Verification items for the finished model (mm, model axes). Face numbers are marked on the shaded views. A direction names the side the tool comes from. Give positions to 0.01 mm unless a question says otherwise; leave off trailing zeros. Loops run counter-clockwise (first coordinate to the right, second up) from the corner with the lowest first, then second, coordinate; pieces in that order, holes last. Notation, with made-up numbers: (43.25, -31.75) - (72.25, -31.75) arc R25 ccw to (72.25, 7.25) - close; hole circle Ø10 at (-8, -1). An arc over 180 degrees is marked (long way). Answer in a Markdown table with one row per item.
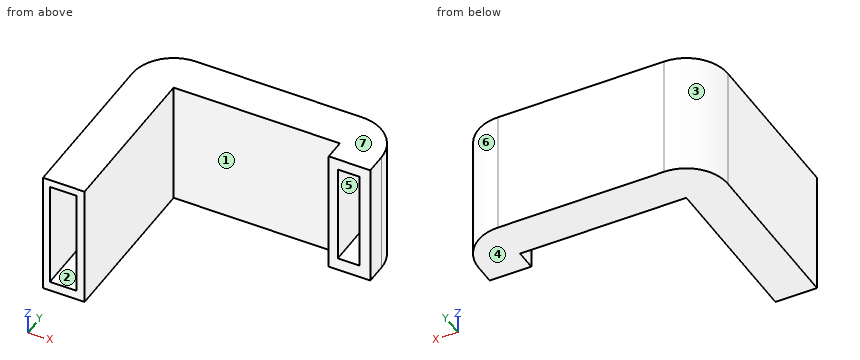
```python
from build123d import *

# Parameters (mm, degrees)
EXTRU_MINCE3_DEPTH      = 30
ESQUISSE9_W             = 6.386782908
ESQUISSE9_H             = 25.842816024
ENL_V_MAT_EXTRU_1_DEPTH = 40
ESQUISSE10_W            = 5.204045332
ESQUISSE10_H            = 24.186983419
ENL_V_MAT_EXTRU_2_DEPTH = 10


with BuildPart() as part:
    # Esquisse5 → Extru.-Mince3 (new body)
    with BuildSketch(Plane.XY):
        with BuildLine():
            Line((-30, -50), (-30, -10))
            ThreePointArc((-30, -10), (-27.071067812, -2.928932188), (-20, 0))
            Line((-20, 0), (20, 0))
            ThreePointArc((20, 0), (27.071067812, -2.928932188), (30, -10))
            Line((30, -10), (30, -15))
            Line((30, -15), (20, -15))
            Line((20, -15), (20, -10))
            Line((20, -10), (-20, -10))
            Line((-20, -10), (-20, -50))
            Line((-20, -50), (-30, -50))
        make_face()
    extrude(amount=EXTRU_MINCE3_DEPTH)

    # Esquisse9 → Enlèv. mat.-Extru.1 (cut)
    with BuildSketch(Plane.XZ.offset(50)):
        with Locations((-25.133173479, 15.236547515)):
            Rectangle(ESQUISSE9_W, ESQUISSE9_H)
    extrude(amount=-ENL_V_MAT_EXTRU_1_DEPTH, mode=Mode.SUBTRACT)

    # Esquisse10 → Enlèv. mat.-Extru.2 (cut)
    with BuildSketch(Plane.XZ.offset(15)):
        with Locations((24.778352206, 15.177410637)):
            Rectangle(ESQUISSE10_W, ESQUISSE10_H)
    extrude(amount=-ENL_V_MAT_EXTRU_2_DEPTH, mode=Mode.SUBTRACT)


solid = part.part
```
Q1. Sectioned sample at A-A (y = -17). Record the cut outline in (x, z), and give its area (3 significant figures).
Completed:
| item | result |
|---|---|
| outline | (-30, 0) - (-20, 0) - (-20, 30) - (-30, 30) - close; hole (-28.33, 2.32) - (-21.94, 2.32) - (-21.94, 28.16) - (-28.33, 28.16) - close |
| area | 135 mm^2 |
Q2. Sectioned sample at C-C (x = -25). Record the cut outline in (y, z).
Completed:
| item | result |
|---|---|
| outline | (-50, 0) - (-1.34, 0) - (-1.34, 30) - (-50, 30) - (-50, 28.16) - (-10, 28.16) - (-10, 2.32) - (-50, 2.32) - close |
Q3. Sectioned sample at D-D (y = -6.5). Record the cut outline in (x, z), and give its area (3 significant figures).
Completed:
| item | result |
|---|---|
| outline | (-29.37, 0) - (29.37, 0) - (29.37, 30) - (-29.37, 30) - close; hole (22.18, 3.08) - (27.38, 3.08) - (27.38, 27.27) - (22.18, 27.27) - close |
| area | 1,640 mm^2 |
Q4. Sectioned sample at B-B (z = 14.25). Record the cut outline in (x, y).
Completed:
| item | result |
|---|---|
| outline | (-30, -50) - (-28.33, -50) - (-28.33, -10) - (-21.94, -10) - (-21.94, -50) - (-20, -50) - (-20, -10) - (20, -10) - (20, -15) - (22.18, -15) - (22.18, -5) - (27.38, -5) - (27.38, -15) - (30, -15) - (30, -10) arc R10 ccw to (20, 0) - (-20, 0) arc R10 ccw to (-30, -10) - close |
Q5. Go/stop test with flat-tipped pins: P1, Ø15, axis at x = -2, z = 22, coming from the -Y side; P2, Ø10, axis at y = -29, z = 19.5, coming from the +X side; P3, Ø1.6, axis at x = 25, z = 11.5, coming from the -Y side. Record where each tip stops, or that it passes through.
Completed:
| item | result |
|---|---|
| P1 | y = -10 |
| P2 | x = -20 |
| P3 | y = -5 |
Q6. Draft check along Z on the marked faces 4, 5, 6 and 7. Enter one of: +Z half, -Z half, draft (parallel to the pull), parting line (faces both ways), or undercut.
Completed:
| item | result |
|---|---|
| face 4 | -Z half |
| face 5 | undercut |
| face 6 | draft |
| face 7 | +Z half |
Q7. Tool access check on the marked faces 1, 2 and 3. Record the directions out of +Z, -Z, +X, -X, +Y, -Y that give a thin tool (end or side, any length) a straight path to the whole face; none if there is none.
Completed:
| item | result |
|---|---|
| face 1 | +Z, -Z, -Y |
| face 2 | -Y |
| face 3 | +Z, -Z, -X, +Y |
Q8. Thickness scan on line 1 (X direction, y = -11.5, z = 10); line 2 (X direction, y = -47, z = 13.25); line 3 (Z direction, x = -22, y = -37). Record the ranges inside material, lowest first.
Completed:
| item | result |
|---|---|
| line 1 | -30 to -28.33, -21.94 to -20, 20 to 22.18, 27.38 to 30 |
| line 2 | -30 to -28.33, -21.94 to -20 |
| line 3 | 0 to 2.32, 28.16 to 30 |
